Check sheet for the modelled part. Datum: model origin and axes. Units: mm. A direction names the side the tool comes from. Round coordinates to 2 decimals unless told otherwise and drop trailing zeros. Loops run counter-clockwise (first coordinate to the right, second up) from the corner with the lowest first, then second, coordinate; pieces in that order, holes last. Notation, with made-up numbers: (-4, -10) -> (1, -10) arc R16 cw to (1, 7) -> close; hole circle Ø8 at (-30, 69). An arc over 180 degrees is marked (long way). Return JSON: item names as keys, results as strings.
from build123d import *

# Parameters (mm, degrees)
F0_R          = 6
F1_DEPTH      = 10
F2_R          = 10
F3_DEPTH      = 8
F3_DEPTH_BACK = 8


with BuildPart() as f1:
    # F0 (on Top) → F1 (new body)
    with BuildSketch(Plane.XY):
        with BuildLine():
            add(Edge.make_bspline(
                [(15.035214282, 35.7758070535), (20.6547243447, 29.9096895942), (32.0572190076, 19.3354156229), (43.3709472389, 18.3830413599), (50.0389123718, 17.9999579396)],
                knots=[0.1100015048, 0.1100015048, 0.1100015048, 0.1100015048, 0.5520103315, 1, 1, 1, 1], degree=3))
            add(Edge.make_bspline(
                [(10.8487541415, 40.2425303512), (12.240880162, 38.7336352898), (13.6367024745, 37.2356913565), (15.035214282, 35.7758070535)],
                knots=[0, 0, 0, 0, 0.1100015048, 0.1100015048, 0.1100015048, 0.1100015048], degree=3))
            ThreePointArc((10.8487541415, 40.2425303512), (-8.0225440308, 41.9925361174), (-18, 25.8792252449))
            Line((-18, 25.8792252449), (-18, -24.1207747551))
            ThreePointArc((-18, -24.1207747551), (-7.1750439774, -40.6289165015), (12.2798604358, -37.281512868))
            add(Edge.make_bspline(
                [(12.2798604358, -37.281512868), (12.6087941785, -36.9495490353), (12.9376997677, -36.6175538258), (13.266753224, -36.2860227548)],
                knots=[0, 0, 0, 0, 0.030015942, 0.030015942, 0.030015942, 0.030015942], degree=3))
            add(Edge.make_bspline(
                [(13.266753224, -36.2860227548), (18.573084972, -30.9397368732), (29.2837115537, -20.4679750546), (43.1130211826, -18.8256033287), (50.0389123718, -17.9999579396)],
                knots=[0.030015942, 0.030015942, 0.030015942, 0.030015942, 0.5140544551, 1, 1, 1, 1], degree=3))
            ThreePointArc((50.0389123718, -17.9999579396), (68, 0), (50.0389123718, 17.9999579396))
        make_face()
        with Locations((0, -24.1207747551)):
            Circle(F0_R, mode=Mode.SUBTRACT)
        with Locations((50, 0)):
            Circle(F0_R, mode=Mode.SUBTRACT)
        with Locations((0, 25.8792252449)):
            Circle(F0_R, mode=Mode.SUBTRACT)
    extrude(amount=F1_DEPTH)

    # F2 (on Front) → F3 (join, two sides)
    with BuildSketch(Plane.XZ) as f3_sk:
        with BuildLine():
            Line((-70, 0), (40, 0))
            Line((40, 0), (40, 10))
            add(Edge.make_bspline(
                [(-54.1361760858, 37.2426733488), (-45.1191100189, 30.1758346752), (-14.9531909541, 16.7242072459), (16.1924294121, 11.4815951801), (40, 10)],
                knots=[0.0529916149, 0.0529916149, 0.0529916149, 0.0529916149, 0.4594202582, 1, 1, 1, 1], degree=3))
            add(Edge.make_bspline(
                [(-57.4545068819, 40.0723712452), (-56.4207333208, 39.1074668132), (-55.3118532927, 38.1640729584), (-54.1361760858, 37.2426733488)],
                knots=[0, 0, 0, 0, 0.0529916149, 0.0529916149, 0.0529916149, 0.0529916149], degree=3))
            ThreePointArc((-57.4545068819, 40.0723712452), (-90.9951442886, 28.5729686066), (-70, 0))
        make_face()
        with Locations((-70, 22)):
            Circle(F2_R, mode=Mode.SUBTRACT)
    extrude(amount=F3_DEPTH)
    extrude(f3_sk.sketch, amount=-F3_DEPTH_BACK)


solid = f1.part
Q1. Section check B-B (y = -11.5). Record the boundary of the cut face in (x, z), then the cut area to 3 significant figures.
Results list:
{"outline": "(-18, 0) -> (63.85, 0) -> (63.85, 10) -> (-18, 10) -> close", "area": "818 mm^2"}
Q2. Go/stop test with flat-tipped pins: pin 1 (5 mm diameter, centred on y = 3.5, z = 28.5, fed in from -X); pin 2 (3 mm diameter, centred on y = -13, z = 3.5, fed in from -X); pin 3 (10 mm diameter, centred on y = 3.5, z = 30, fed in from -X). Record where each tip stops, or that it passes through.
Results list:
{"pin 1": "x = -91.63", "pin 2": "x = -18", "pin 3": "x = -91.79"}
Q3. Section check A-A (z = 8.5). Count the separate pieces of the cut face and the enclosed holes in it, then the cut area to 3 significant figures.
Results list:
{"separate pieces": "1", "enclosed holes": "3", "area": "5,540 mm^2"}
Q4. Tool access check on faces 5 (the flat face through (-18, 17, 5)), 6 (the flat face through (-18, -16, 5)), 7 (the flat face through (13, 0, 0)). Record the directions out of +Z, -Z, +X, -X, +Y, -Y that give a thin tool (end or side, any length) a straight path to the whole face; none if there is none.
Results list:
{"face 5": "+Z, -Z, -X, +Y", "face 6": "+Z, -Z, -X, -Y", "face 7": "-Z, +X, -X, +Y, -Y"}
Q5. Draft check along Y on faces 1 (the cylindrical face through (44, 0, 5)), 2 (the cylindrical face through (-7.44, -40.51, 4.93)), 3 (the cylindrical face through (-90.815, -0.112, 29.122)), 4 (the cylindrical face through (-1.3, 20.02, 4.93)). Enter one of: released by +Y, released by -Y, zero draft, split by the parting line, or undercut.
Results list:
{"face 1": "undercut", "face 2": "released by -Y", "face 3": "zero draft", "face 4": "undercut"}
Q6. Material ranges on line 1 (Y direction, x = 0, z = 8.25); line 2 (Y direction, x = 50, z = 6.5); line 3 (Z direction, x = -70, y = -1), recorded low to high.
Results list:
{"line 1": "-42.12 to -30.12, -18.12 to 19.88, 31.88 to 43.88", "line 2": "-18 to -6, 6 to 18", "line 3": "0 to 12, 32 to 44"}
